from build123d import *

# Parameters (mm, degrees)
F0_W     = 176
F0_H     = 26
F0_W_2   = 170
F0_H_2   = 20
F0_W_3   = 200
F0_H_3   = 50
F1_DEPTH = 2
F2_DEPTH = 8.5
F3_R     = 5
F4_R     = 5


with BuildPart() as f1:
    # F0 (on Top) → F1 (new body)
    with BuildSketch(Plane.XY):
        Rectangle(F0_W, F0_H)
        Rectangle(F0_W_2, F0_H_2, mode=Mode.SUBTRACT)
        Rectangle(F0_W_3, F0_H_3)
        Rectangle(F0_W, F0_H, mode=Mode.SUBTRACT)
    extrude(amount=F1_DEPTH)

    # F0 (on Top) → F2 (join)
    with BuildSketch(Plane.XY):
        Rectangle(F0_W, F0_H)
        Rectangle(F0_W_2, F0_H_2, mode=Mode.SUBTRACT)
    extrude(amount=F2_DEPTH)

    # F3
    f3_edges = [f1.edges().sort_by_distance(p)[0] for p in [
        (-85, -10, 4.25),
        (-85, 10, 4.25),
        (85, -10, 4.25),
        (85, 10, 4.25),
    ]]
    fillet(f3_edges, radius=F3_R)

    # F4
    f4_edges = [f1.edges().sort_by_distance(p)[0] for p in [
        (0, -10, 0),
    ]]
    fillet(f4_edges, radius=F4_R)


solid = f1.part
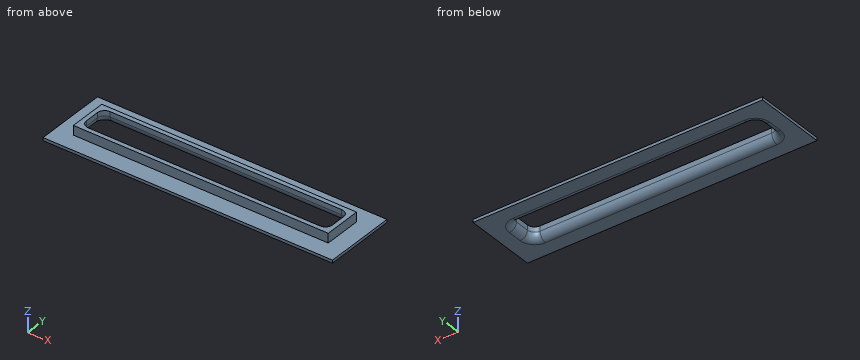
Input: part model. Units: mm. Frame: model coordinates. Coordinates: 2 decimals unless noted, no trailing zeros. Loops run counter-clockwise (first coordinate to the right, second up) from the corner with the lowest first, then second, coordinate; pieces in that order, holes last. Notation, with made-up numbers: (58, 11.25) -> (83, 11.25) arc R8 ccw to (83, 24.25) -> close; hole circle Ø10 at (-12, 15.25). An arc over 180 degrees is marked (long way). One line per item, written item: value.
(1) Pin query (flat end, axial travel): pin 1 Ø1.8 at (y, z) = (-0.5, 6.5) entering from +X; pin 2 Ø3 at (x, y) = (44, 18) entering from +Z; pin 3 Ø3 at (x, y) = (-13, 7.5) entering from -Z; pin 4 Ø2 at (y, z) = (-6.5, 4) entering from -X. Return the tip coordinate at first contact, or that it passes through.
Answer below:
pin 1: stops at x = 88
pin 2: stops at z = 2
pin 3: passes through
pin 4: stops at x = -88
(2) Cut plane A-A (y = -2.5). Output: boundary loops of the cut face in (x, z), then the cut area to 3 significant figures.
Answer below:
outline: (-100, 0) -> (-90, 0) arc R5 ccw to (-85, 5) -> (-85, 8.5) -> (-88, 8.5) -> (-88, 2) -> (-100, 2) -> close; (85, 5) arc R5 ccw to (90, 0) -> (100, 0) -> (100, 2) -> (88, 2) -> (88, 8.5) -> (85, 8.5) -> close
area: 88.3 mm2
(3) Cut plane C-C (z = 6.5). Output: boundary loops of the cut face in (x, y).
Answer below:
outline: (-88, -13) -> (88, -13) -> (88, 13) -> (-88, 13) -> close; hole (-85, -5) arc R5 ccw to (-80, -10) -> (80, -10) arc R5 ccw to (85, -5) -> (85, 5) arc R5 ccw to (80, 10) -> (-80, 10) arc R5 ccw to (-85, 5) -> close
(4) Cut plane B-B (x = -74). Output: boundary loops of the cut face in (y, z), then the cut area to 3 significant figures.
Answer below:
outline: (-25, 0) -> (-15, 0) arc R5 ccw to (-10, 5) -> (-10, 8.5) -> (-13, 8.5) -> (-13, 2) -> (-25, 2) -> close; (10, 5) arc R5 ccw to (15, 0) -> (25, 0) -> (25, 2) -> (13, 2) -> (13, 8.5) -> (10, 8.5) -> close
area: 88.3 mm2
(5) Ray query, line 1 along Y through (x, z) = (53.5, 5.75); line 2 along X through (y, z) = (11.5, 4.75); line 3 along Z through (x, y) = (28.5, -21.5). Return the intervals inside material, ascending.
Answer below:
line 1: y = -13 to -10, 10 to 13
line 2: x = -88 to 88
line 3: z = 0 to 2
